Design review of the part built by this model. Coordinates are the model's own, in mm. Give positions to 0.01 mm unless a question says otherwise; leave off trailing zeros. Loops run counter-clockwise (first coordinate to the right, second up) from the corner with the lowest first, then second, coordinate; pieces in that order, holes last. Notation, with made-up numbers: (55.25, -1.5) - (74.25, -1.5) arc R17 ccw to (74.25, 16.5) - close; hole circle Ø7 at (35.5, 61.5). An arc over 180 degrees is marked (long way). Put each result on its own line as item: value. Start each with the question number.
```python
from build123d import *

# Parameters (mm, degrees)
SKETCH1_R           = 1.55
SKETCH1_R_2         = 12.5
BOSS_EXTRUDE1_DEPTH = 1.6


with BuildPart() as part:
    # Sketch1 → Boss-Extrude1 (new body)
    with BuildSketch(Plane.XY):
        Polygon((-34.951905284, 37.5), (34.951905284, 37.5), (49.951905284, 11.519237886), (15, -49.019237886), (-15, -49.019237886), (-49.951905284, 11.519237886), align=None)
        with Locations((-30, 27.5)):
            Circle(SKETCH1_R, mode=Mode.SUBTRACT)
        with Locations((30, 27.5)):
            Circle(SKETCH1_R, mode=Mode.SUBTRACT)
        with Locations((38.815698604, 12.230762114)):
            Circle(SKETCH1_R, mode=Mode.SUBTRACT)
        with Locations((8.815698604, -39.730762114)):
            Circle(SKETCH1_R, mode=Mode.SUBTRACT)
        with Locations((-8.815698604, -39.730762114)):
            Circle(SKETCH1_R, mode=Mode.SUBTRACT)
        with Locations((-38.815698604, 12.230762114)):
            Circle(SKETCH1_R, mode=Mode.SUBTRACT)
        Circle(SKETCH1_R_2, mode=Mode.SUBTRACT)
    extrude(amount=BOSS_EXTRUDE1_DEPTH)


solid = part.part
```
Item 1: Consider section C-C (z = 1.3). State the section outline as (x, y) points.
Item 2: Consider section D-D (y = 27.5). State the section outline as (x, z) points.
Item 3: Consider section B-B (y = 0). State the section outline as (x, z) points.
Item 4: Mouldability with a two-part tool opening along Y and no side actions: class faces 1 (the cylindrical face through (-29.17, 28.81, 0.79)), 2 (the cylindrical face through (-9.958, -38.683, 0.789)), 3 (the flat face through (-42.557, 24.328, 0.789)), 4 (the flat face through (-32.231, -19.174, 0.789)) as pulls with the +Y half, pulls with the -Y half, needs draft (parallel to the pull), parting line crosses it, or undercut.
Item 5: Consider section A-A (x = 0.5). State the section outline as (y, z) points, plus the area to 3 significant figures.
Item 6: For L1, parallel to Y at x = 38, z = 0.15; L2, parallel to Y at x = 10, z = 1.4; L3, parallel to Y at x = -38.5, z = 0.9, list the stretches that pass through material, from the lowest coordinate up. Write a range as from..to.
Geometry says:
1. outline: (-49.95, 11.52) - (-15, -49.02) - (15, -49.02) - (49.95, 11.52) - (34.95, 37.5) - (-34.95, 37.5) - close; hole circle Ø3.1 at (-38.82, 12.23); hole circle Ø3.1 at (-30, 27.5); hole circle Ø25 at (0, 0); hole circle Ø3.1 at (-8.82, -39.73); hole circle Ø3.1 at (8.82, -39.73); hole circle Ø3.1 at (30, 27.5); hole circle Ø3.1 at (38.82, 12.23)
2. outline: (-40.73, 0) - (-31.55, 0) - (-31.55, 1.6) - (-40.73, 1.6) - close; (-28.45, 0) - (28.45, 0) - (28.45, 1.6) - (-28.45, 1.6) - close; (31.55, 0) - (40.73, 0) - (40.73, 1.6) - (31.55, 1.6) - close
3. outline: (-43.3, 0) - (-12.5, 0) - (-12.5, 1.6) - (-43.3, 1.6) - close; (12.5, 0) - (43.3, 0) - (43.3, 1.6) - (12.5, 1.6) - close
4. face 1: undercut
4. face 2: undercut
4. face 3: pulls with the +Y half
4. face 4: pulls with the -Y half
5. outline: (-49.02, 0) - (-12.49, 0) - (-12.49, 1.6) - (-49.02, 1.6) - close; (12.49, 0) - (37.5, 0) - (37.5, 1.6) - (12.49, 1.6) - close
5. area: 98.5 mm2
6. L1: y = -9.18..10.91, 13.55..32.22
6. L2: y = -49.02..-40.73, -38.73..-7.5, 7.5..37.5
6. L3: y = -8.32..10.71, 13.75..31.35
